Autodesk Inventor part; units mm, degrees
ref_plane "YZ Plane" through (0, 0, 0) normal (1, 0, 0) x (0, 1, 0)
ref_plane "XZ Plane" through (0, 0, 0) normal (0, 1, 0) x (-1, 0, 0)
ref_plane "XY Plane" through (0, 0, 0) normal (0, 0, 1) x (1, 0, 0)
sketch "Sketch1" plane through (0, 0, 0) normal (0, 0, 1) x (1, 0, 0)
  line L0 (8.2, 0) -> (0, 0)
  line L1 (8.6, 0.4) -> (8.2, 0)
  line L2 (8.6, 3.502) -> (8.6, 0.4)
  arc A0 (8.6, 3.502) -> (8.531, 3.6168) centre (8.47, 3.502) ccw
  arc A1 (8.1612, 3.9682) -> (8.531, 3.6168) centre (8.9765, 4.4558) ccw
  arc A2 (8.1612, 3.9682) -> (8.0496, 4.0315) centre (8.0496, 3.9015) ccw
  line L3 (7.7695, 4.0315) -> (8.0496, 4.0315)
  arc A3 (7.7695, 4.8802) -> (7.7695, 4.0315) centre (7.6197, 4.4558) ccw
  line L4 (8.0496, 4.8802) -> (7.7695, 4.8802)
  arc A4 (8.0496, 4.8802) -> (8.1612, 4.9434) centre (8.0496, 5.0102) ccw
  arc A5 (8.531, 5.2949) -> (8.1612, 4.9434) centre (8.9765, 4.4558) ccw
  arc A6 (8.531, 5.2949) -> (8.6, 5.4097) centre (8.47, 5.4097) ccw
  line L5 (8.6, 6.0117) -> (8.6, 5.4097)
  line L6 (8.2, 6.5) -> (8.6, 6.0117)
  line L7 (0, 6.5) -> (8.2, 6.5)
  line L8 (-0.4, 6.0117) -> (0, 6.5)
  line L9 (-0.4, 5.4097) -> (-0.4, 6.0117)
  arc A7 (-0.4, 5.4097) -> (-0.331, 5.2949) centre (-0.27, 5.4097) ccw
  arc A8 (0.0388, 4.9434) -> (-0.331, 5.2949) centre (-0.7765, 4.4558) ccw
  arc A9 (0.0388, 4.9434) -> (0.1504, 4.8802) centre (0.1504, 5.0102) ccw
  line L10 (0.4305, 4.8802) -> (0.1504, 4.8802)
  arc A10 (0.4305, 4.0315) -> (0.4305, 4.8802) centre (0.5803, 4.4558) ccw
  line L11 (0.1504, 4.0315) -> (0.4305, 4.0315)
  arc A11 (0.1504, 4.0315) -> (0.0388, 3.9682) centre (0.1504, 3.9015) ccw
  arc A12 (-0.331, 3.6168) -> (0.0388, 3.9682) centre (-0.7765, 4.4558) ccw
  arc A13 (-0.331, 3.6168) -> (-0.4, 3.502) centre (-0.27, 3.502) ccw
  line L12 (-0.4, 0.4) -> (-0.4, 3.502)
  line L13 (0, 0) -> (-0.4, 0.4)
  point P0 (4.1, 0)
extrude "Extrusion1" add sketch "Sketch1" along normal blind 42
sketch "Sketch2" plane through (0, 6.5, 0) normal (0, 1, 0) x (1, 0, 0)
  circle A0 centre (4.1, -4) radius 2
  circle A1 centre (4.1, -38) radius 2
  line L0 (8.2, 0) -> (0, 0)
  line L1 (4.1, 0) -> (4.1, -42)
  line L2 (8.2, -42) -> (0, -42)
  dimension "d2" = 4
  dimension "d3" = 4
  dimension "d4" = 4
  dimension "d5" = 4
extrude "Extrusion2" cut sketch "Sketch2" against normal blind 10
properties part number "mgn9_carriage_holder"
Verification items for the finished model (mm, model axes). Give positions to 0.01 mm unless a question says otherwise; leave off trailing zeros. Order: outer loops, then holes, each group sorted by start corner. A loop starts at its lowest first (then second) coordinate and runs counter-clockwise, first axis right, second up. Notation, with made-up numbers: (37, 27) -> (87, 27) arc R7 ccw to (87, 39) -> close; hole circle Ø3 at (75, 52.5). An arc over 180 degrees is marked (long way). One line per item, written item: value.
(1) Sectioned sample at C-C on y = 1. Record the cut outline in (x, z).
Final values:
outline: (-0.4, 0) -> (8.6, 0) -> (8.6, 42) -> (-0.4, 42) -> close; hole circle Ø4 at (4.1, 4); hole circle Ø4 at (4.1, 38)
(2) Draft check along X on faces 1 (the face through (8.6, 2, 21)), 2 (the face through (1.03, 4.47, 20.71)), 3 (the face through (4, 6.5, 21)). Enter one of: pulls with the +X half, pulls with the -X half, needs draft (parallel to the pull), parting line crosses it, or undercut.
Final values:
face 1: pulls with the +X half
face 2: undercut
face 3: needs draft
(3) Sectioned sample at B-B on x = 4.1. Record the cut outline in (y, z), then the cut area to 3 significant figures.
Final values:
outline: (0, 0) -> (6.5, 0) -> (6.5, 2) -> (0, 2) -> close; (0, 6) -> (6.5, 6) -> (6.5, 36) -> (0, 36) -> close; (0, 40) -> (6.5, 40) -> (6.5, 42) -> (0, 42) -> close
area: 221 mm^2
(4) Scan lines: line 1 along Z through (x, y) = (4.1, 2); line 2 along Y through (x, z) = (7.5, 28); line 3 along Z through (x, y) = (2.5, 5). Record each from-to range of solid material in increasing order. Write a range as [from, to].
Final values:
line 1: [0, 2], [6, 36], [40, 42]
line 2: [0, 4.02], [4.89, 6.5]
line 3: [0, 2.8], [5.2, 36.8], [39.2, 42]
(5) Sectioned sample at D-D on y = 4.5. Record the cut outline in (x, z).
Final values:
outline: (1.03, 0) -> (7.17, 0) -> (7.17, 42) -> (1.03, 42) -> close; hole circle Ø4 at (4.1, 4); hole circle Ø4 at (4.1, 38)
